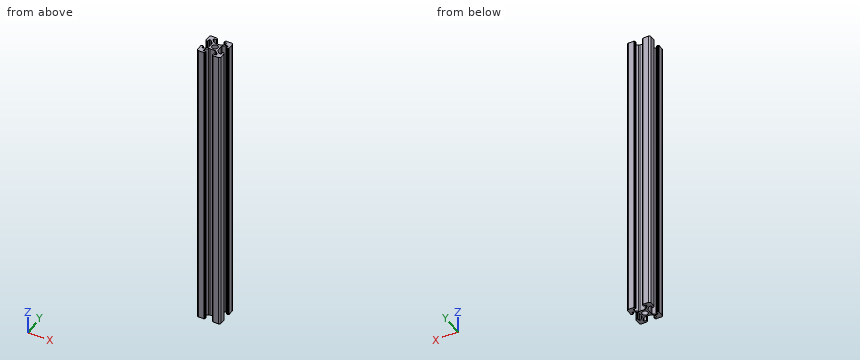
from build123d import *

# Parameters (mm, degrees)
SKETCH_1_R      = 2.5
EXTRUDE_1_DEPTH = 254


with BuildPart() as part:
    # 草图1 → 凸台-拉伸1 (new body)
    with BuildSketch(Plane.XY):
        with BuildLine():
            Line((-8.502261885, -10.002261885), (-3.85, -10.002261885))
            ThreePointArc((-3.85, -10.002261885), (-3.673223305, -9.929038581), (-3.6, -9.752261885))
            Line((-3.6, -9.752261885), (-3.6, -9.502261885))
            Line((-3.6, -9.502261885), (-3.35, -9.502261885))
            ThreePointArc((-3.35, -9.502261885), (-3.173223305, -9.429038581), (-3.1, -9.252261885))
            Line((-3.1, -9.252261885), (-3.1, -8.45))
            ThreePointArc((-3.1, -8.45), (-3.173223305, -8.273223305), (-3.35, -8.2))
            Line((-3.35, -8.2), (-5.25, -8.2))
            ThreePointArc((-5.25, -8.2), (-5.426776695, -8.126776695), (-5.5, -7.95))
            Line((-5.5, -7.95), (-5.5, -6.664213562))
            ThreePointArc((-5.5, -6.664213562), (-5.480969883, -6.568542704), (-5.426776695, -6.487436867))
            Line((-5.426776695, -6.487436867), (-3.278679656, -4.339339828))
            ThreePointArc((-3.278679656, -4.339339828), (-2.792044633, -4.014180701), (-2.218019485, -3.9))
            Line((-2.218019485, -3.9), (2.218019485, -3.9))
            ThreePointArc((2.218019485, -3.9), (2.792044633, -4.014180701), (3.278679656, -4.339339828))
            Line((3.278679656, -4.339339828), (5.426776695, -6.487436867))
            ThreePointArc((5.426776695, -6.487436867), (5.480969883, -6.568542704), (5.5, -6.664213562))
            Line((5.5, -6.664213562), (5.5, -7.95))
            ThreePointArc((5.5, -7.95), (5.426776695, -8.126776695), (5.25, -8.2))
            Line((5.25, -8.2), (3.35, -8.2))
            ThreePointArc((3.35, -8.2), (3.173223305, -8.273223305), (3.1, -8.45))
            Line((3.1, -8.45), (3.1, -9.252261885))
            ThreePointArc((3.1, -9.252261885), (3.173223305, -9.429038581), (3.35, -9.502261885))
            Line((3.35, -9.502261885), (3.6, -9.502261885))
            Line((3.6, -9.502261885), (3.6, -9.752261885))
            ThreePointArc((3.6, -9.752261885), (3.673223305, -9.929038581), (3.85, -10.002261885))
            Line((3.85, -10.002261885), (8.502261885, -10.002261885))
            ThreePointArc((8.502261885, -10.002261885), (9.562922057, -9.562922057), (10.002261885, -8.502261885))
            Line((10.002261885, -8.502261885), (10.002261885, -3.85))
            ThreePointArc((10.002261885, -3.85), (9.929038581, -3.673223305), (9.752261885, -3.6))
            Line((9.752261885, -3.6), (9.502261885, -3.6))
            Line((9.502261885, -3.6), (9.502261885, -3.35))
            ThreePointArc((9.502261885, -3.35), (9.429038581, -3.173223305), (9.252261885, -3.1))
            Line((9.252261885, -3.1), (8.45, -3.1))
            ThreePointArc((8.45, -3.1), (8.273223305, -3.173223305), (8.2, -3.35))
            Line((8.2, -3.35), (8.2, -5.25))
            ThreePointArc((8.2, -5.25), (8.126776695, -5.426776695), (7.95, -5.5))
            Line((7.95, -5.5), (6.664213562, -5.5))
            ThreePointArc((6.664213562, -5.5), (6.568542704, -5.480969883), (6.487436867, -5.426776695))
            Line((6.487436867, -5.426776695), (4.339339828, -3.278679656))
            ThreePointArc((4.339339828, -3.278679656), (4.014180701, -2.792044633), (3.9, -2.218019485))
            Line((3.9, -2.218019485), (3.9, 2.218019485))
            ThreePointArc((3.9, 2.218019485), (4.014180701, 2.792044633), (4.339339828, 3.278679656))
            Line((4.339339828, 3.278679656), (6.487436867, 5.426776695))
            ThreePointArc((6.487436867, 5.426776695), (6.568542704, 5.480969883), (6.664213562, 5.5))
            Line((6.664213562, 5.5), (7.95, 5.5))
            ThreePointArc((7.95, 5.5), (8.126776695, 5.426776695), (8.2, 5.25))
            Line((8.2, 5.25), (8.2, 3.35))
            ThreePointArc((8.2, 3.35), (8.273223305, 3.173223305), (8.45, 3.1))
            Line((8.45, 3.1), (9.252261885, 3.1))
            ThreePointArc((9.252261885, 3.1), (9.429038581, 3.173223305), (9.502261885, 3.35))
            Line((9.502261885, 3.35), (9.502261885, 3.6))
            Line((9.502261885, 3.6), (9.752261885, 3.6))
            ThreePointArc((9.752261885, 3.6), (9.929038581, 3.673223305), (10.002261885, 3.85))
            Line((10.002261885, 3.85), (10.002261885, 8.502261885))
            ThreePointArc((10.002261885, 8.502261885), (9.562922057, 9.562922057), (8.502261885, 10.002261885))
            Line((8.502261885, 10.002261885), (3.85, 10.002261885))
            ThreePointArc((3.85, 10.002261885), (3.673223305, 9.929038581), (3.6, 9.752261885))
            Line((3.6, 9.752261885), (3.6, 9.502261885))
            Line((3.6, 9.502261885), (3.35, 9.502261885))
            ThreePointArc((3.35, 9.502261885), (3.173223305, 9.429038581), (3.1, 9.252261885))
            Line((3.1, 9.252261885), (3.1, 8.45))
            ThreePointArc((3.1, 8.45), (3.173223305, 8.273223305), (3.35, 8.2))
            Line((3.35, 8.2), (5.25, 8.2))
            ThreePointArc((5.25, 8.2), (5.426776695, 8.126776695), (5.5, 7.95))
            Line((5.5, 7.95), (5.5, 6.664213562))
            ThreePointArc((5.5, 6.664213562), (5.480969883, 6.568542704), (5.426776695, 6.487436867))
            Line((5.426776695, 6.487436867), (3.278679656, 4.339339828))
            ThreePointArc((3.278679656, 4.339339828), (2.792044633, 4.014180701), (2.218019485, 3.9))
            Line((2.218019485, 3.9), (-2.218019485, 3.9))
            ThreePointArc((-2.218019485, 3.9), (-2.792044633, 4.014180701), (-3.278679656, 4.339339828))
            Line((-3.278679656, 4.339339828), (-5.426776695, 6.487436867))
            ThreePointArc((-5.426776695, 6.487436867), (-5.480969883, 6.568542704), (-5.5, 6.664213562))
            Line((-5.5, 6.664213562), (-5.5, 7.95))
            ThreePointArc((-5.5, 7.95), (-5.426776695, 8.126776695), (-5.25, 8.2))
            Line((-5.25, 8.2), (-3.35, 8.2))
            ThreePointArc((-3.35, 8.2), (-3.173223305, 8.273223305), (-3.1, 8.45))
            Line((-3.1, 8.45), (-3.1, 9.252261885))
            ThreePointArc((-3.1, 9.252261885), (-3.173223305, 9.429038581), (-3.35, 9.502261885))
            Line((-3.35, 9.502261885), (-3.6, 9.502261885))
            Line((-3.6, 9.502261885), (-3.6, 9.752261885))
            ThreePointArc((-3.6, 9.752261885), (-3.673223305, 9.929038581), (-3.85, 10.002261885))
            Line((-3.85, 10.002261885), (-8.502261885, 10.002261885))
            ThreePointArc((-8.502261885, 10.002261885), (-9.562922057, 9.562922057), (-10.002261885, 8.502261885))
            Line((-10.002261885, 8.502261885), (-10.002261885, 3.85))
            ThreePointArc((-10.002261885, 3.85), (-9.929038581, 3.673223305), (-9.752261885, 3.6))
            Line((-9.752261885, 3.6), (-9.502261885, 3.6))
            Line((-9.502261885, 3.6), (-9.502261885, 3.35))
            ThreePointArc((-9.502261885, 3.35), (-9.429038581, 3.173223305), (-9.252261885, 3.1))
            Line((-9.252261885, 3.1), (-8.45, 3.1))
            ThreePointArc((-8.45, 3.1), (-8.273223305, 3.173223305), (-8.2, 3.35))
            Line((-8.2, 3.35), (-8.2, 5.25))
            ThreePointArc((-8.2, 5.25), (-8.126776695, 5.426776695), (-7.95, 5.5))
            Line((-7.95, 5.5), (-6.664213562, 5.5))
            ThreePointArc((-6.664213562, 5.5), (-6.568542704, 5.480969883), (-6.487436867, 5.426776695))
            Line((-6.487436867, 5.426776695), (-4.339339828, 3.278679656))
            ThreePointArc((-4.339339828, 3.278679656), (-4.014180701, 2.792044633), (-3.9, 2.218019485))
            Line((-3.9, 2.218019485), (-3.9, -2.218019485))
            ThreePointArc((-3.9, -2.218019485), (-4.014180701, -2.792044633), (-4.339339828, -3.278679656))
            Line((-4.339339828, -3.278679656), (-6.487436867, -5.426776695))
            ThreePointArc((-6.487436867, -5.426776695), (-6.568542704, -5.480969883), (-6.664213562, -5.5))
            Line((-6.664213562, -5.5), (-7.95, -5.5))
            ThreePointArc((-7.95, -5.5), (-8.126776695, -5.426776695), (-8.2, -5.25))
            Line((-8.2, -5.25), (-8.2, -3.35))
            ThreePointArc((-8.2, -3.35), (-8.273223305, -3.173223305), (-8.45, -3.1))
            Line((-8.45, -3.1), (-9.252261885, -3.1))
            ThreePointArc((-9.252261885, -3.1), (-9.429038581, -3.173223305), (-9.502261885, -3.35))
            Line((-9.502261885, -3.35), (-9.502261885, -3.6))
            Line((-9.502261885, -3.6), (-9.752261885, -3.6))
            ThreePointArc((-9.752261885, -3.6), (-9.929038581, -3.673223305), (-10.002261885, -3.85))
            Line((-10.002261885, -3.85), (-10.002261885, -8.502261885))
            ThreePointArc((-10.002261885, -8.502261885), (-9.562922057, -9.562922057), (-8.502261885, -10.002261885))
        make_face()
        Circle(SKETCH_1_R, mode=Mode.SUBTRACT)
    extrude(amount=EXTRUDE_1_DEPTH)


solid = part.part
Read the model definition and answer for the solid it produces. Units are mm, in the model's axes. Give positions to 0.01 mm unless a question says otherwise; leave off trailing zeros. Write each loop counter-clockwise with the first axis right and the second up, starting at its lowest first coordinate (ties: lowest second). Pieces come first, ordered by that corner, then holes. Notation, with made-up numbers: (-8, -26) -> (48, -26) arc R12 cw to (48, -21) -> close; hole circle Ø3 at (89.5, -12). An arc over 180 degrees is marked (long way). Answer as a JSON object with one key per item and string values. Group by question number.
1) Each of these flat-tipped pins is pushed along its axis until it touches: P1, Ø1, axis at x = 1, z = 132, coming from the +Y side; P2, Ø1, axis at y = 2.5, z = 107, coming from the -X side; P3, Ø2, axis at y = -0.5, z = 187, coming from the +X side. Where does it stop, or does it pass through?
2) Find section A-A (x = 0). Write down the section's boundary in (y, z), and give its area (3 significant figures).
3) Consider L1, parallel to Y at x = -7, z = 38.5; L2, parallel to X at y = 3.75, z = 98; L3, parallel to Y at x = 0, z = 203. Determine where each line is inside the solid, lowest interval first. Write a range as from..to.
Values follow:
{
 "1": {"P1": "stops at y = 3.9", "P2": "stops at x = -4.12", "P3": "stops at x = 3.9"},
 "2": {"outline": "(-3.9, 0) -> (-2.5, 0) -> (-2.5, 254) -> (-3.9, 254) -> close; (2.5, 0) -> (3.9, 0) -> (3.9, 254) -> (2.5, 254) -> close", "area": "711 mm2"},
 "3": {"L1": "y = -10..-5.5, 5.5..10", "L2": "x = -9.98..-8.2, -4.81..4.81, 8.2..9.98", "L3": "y = -3.9..-2.5, 2.5..3.9"}
}
